from build123d import *

# Parameters (mm, degrees)
SKETCH1_R           = 12.5
SKETCH1_R_2         = 7.5
BOSS_EXTRUDE1_DEPTH = 15
SKETCH1_3_W         = 30
SKETCH1_3_H         = 15
BOSS_EXTRUDE2_DEPTH = 45
BOSS_EXTRUDE3_START = 15
SKETCH1_4_W         = 30
SKETCH1_4_H         = 15
BOSS_EXTRUDE3_DEPTH = 45
CUT_EXTRUDE1_START  = 10
SKETCH3_R           = 6
CUT_EXTRUDE1_DEPTH  = 30


with BuildPart() as part:
    # Sketch1 → Boss-Extrude1 (new body)
    with BuildSketch(Plane(origin=(0, 0, 0), x_dir=(1, 0, 0), z_dir=(0, 1, 0))):
        with BuildLine():
            Line((150, 25), (0, 25))
            ThreePointArc((0, 25), (-25, 0), (0, -25))
            Line((0, -25), (20, -25))
            Line((20, -25), (20, -10))
            Line((20, -10), (50, -10))
            Line((50, -10), (50, -25))
            Line((50, -25), (120, -25))
            Line((120, -25), (150, -25))
            Line((150, -25), (150, 25))
        make_face()
        with Locations(Location((0, 0, 0), (0, 0, 270))):
            Circle(SKETCH1_R, mode=Mode.SUBTRACT)
        with Locations(Location((135, 0, 0), (0, 0, 270))):
            Circle(SKETCH1_R_2, mode=Mode.SUBTRACT)
    extrude(amount=BOSS_EXTRUDE1_DEPTH)

    # Sketch1<3> → Boss-Extrude2 (add)
    with BuildSketch(Plane(origin=(0, 0, 0), x_dir=(1, 0, 0), z_dir=(0, 1, 0))):
        with Locations((35, -17.5)):
            Rectangle(SKETCH1_3_W, SKETCH1_3_H)
    extrude(amount=BOSS_EXTRUDE2_DEPTH)

    # Sketch1<4> → Boss-Extrude3 (add)
    with BuildSketch(Plane(origin=(0, 0, 0), x_dir=(1, 0, 0), z_dir=(0, 1, 0)).offset(BOSS_EXTRUDE3_START)):
        with Locations((135, -32.5)):
            Rectangle(SKETCH1_4_W, SKETCH1_4_H)
    extrude(amount=-BOSS_EXTRUDE3_DEPTH)

    # Sketch3 → Cut-Extrude1 (cut)
    with BuildSketch(Plane.XY.offset(CUT_EXTRUDE1_START)):
        with BuildLine():
            ThreePointArc((35, 45), (45.606601718, 40.606601718), (50, 30))
            Line((50, 30), (50, 45))
            Line((50, 45), (35, 45))
        make_face()
        with BuildLine():
            Line((20, 45), (20, 30))
            ThreePointArc((20, 30), (24.393398282, 40.606601718), (35, 45))
            Line((35, 45), (20, 45))
        make_face()
        with Locations(Location((35, 30, 0), (0, 0, 180))):
            Circle(SKETCH3_R)
        with BuildLine():
            ThreePointArc((150, -15), (135, -30), (120, -15))
            Line((120, -15), (120, -39.427079815))
            Line((120, -39.427079815), (150, -39.427079815))
            Line((150, -39.427079815), (150, -15))
        make_face()
        with Locations(Location((135, -15, 0), (0, 0, 180))):
            Circle(SKETCH3_R)
    extrude(amount=CUT_EXTRUDE1_DEPTH, mode=Mode.SUBTRACT)


solid = part.part
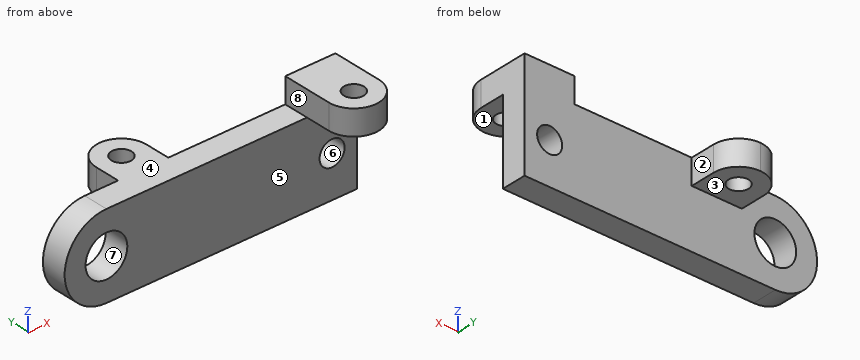
Build history of the part. All positions in model axes, mm. Face numbers are marked on the shaded views. A direction names the side the tool comes from. Round coordinates to 2 decimals unless told otherwise and drop trailing zeros. Write each loop counter-clockwise with the first axis right and the second up, starting at its lowest first coordinate (ties: lowest second). Pieces come first, ordered by that corner, then holes. Notation, with made-up numbers: M -14.75,-6.5 L 44.25,-6.5 A14 cw 44.25,4.5 Z; hole C 68,87.25 d4. An arc over 180 degrees is marked long. Answer as a JSON object with one key per item and string values. Group by question number.
(1) Cut at D-D (z = 19). Give the cut face in (x, y).
(2) Drill centre lines: L1, parallel to X at y = 8, z = 0; L2, parallel to Y at x = 135, z = 36; L3, parallel to X at y = -15, z = 34. Where is each one in solid material? Low to high.
(3) Cut at C-C (y = 8). Give the cut face in (x, z).
(4) Cut at B-B (x = 135). Give the cut face in (y, z), and give its area (3 significant figures).
(5) Which spindle directions (+Z, -Z, +X, -X, +Y, -Y) get a long thin tool onto all of the face, cutting with end or side? Do the marked faces 1, 2, 3 and 4. Say none if no direction does.
(6) Cut at A-A (z = 0). Give the cut face in (x, y).
(7) Mould opens along X. For the marked faces 5, 6, 7 and 8 say: pulls with the +X half, pulls with the -X half, needs draft (parallel to the pull), parting line crosses it, or undercut.
(8) Flat gauge pins, fed straight in: pin 1 (11 mm diameter, centred on x = 35, y = 30, fed in from -Z); pin 2 (5 mm diameter, centred on x = 78, z = 11, fed in from +Y); pin 3 (14 mm diameter, centred on x = 135, y = -15, fed in from +Z); pin 4 (16.5 mm diameter, centred on y = 23.5, z = 14.5, fed in from -X). Where does each tip first touch, or does it go through?
Responses:
{
 "1": {"outline": "M -16.25,0 L 150,0 L 150,15 L 50,15 L 50,30 A15 ccw 20,30 L 20,15 L -16.25,15 Z; hole C 35,30 d12"},
 "2": {"L1": "x = -25 to -12.5, 12.5 to 127.5, 142.5 to 150", "L2": "y = -30 to -21, -9 to 15", "L3": "x = 120 to 129, 141 to 150"},
 "3": {"outline": "M 0,-25 L 150,-25 L 150,40 L 120,40 L 120,25 L 0,25 A25 ccw Z; hole C 0,0 d25; hole C 135,0 d15"},
 "4": {"outline": "M -30,25 L -21,25 L -21,40 L -30,40 Z; M -9,25 L 0,25 L 0,7.5 L 15,7.5 L 15,40 L -9,40 Z; M 0,-25 L 15,-25 L 15,-7.5 L 0,-7.5 Z", "area": "1,020 mm2"},
 "5": {"face 1": "-Z, +X, -X, -Y", "face 2": "+Z, -Z, +X, +Y", "face 3": "-Z, +X, -X, +Y", "face 4": "+Z, -X, +Y, -Y"},
 "6": {"outline": "M -25,0 L -12.5,0 L -12.5,15 L -25,15 Z; M 12.5,0 L 127.5,0 L 127.5,15 L 12.5,15 Z; M 142.5,0 L 150,0 L 150,15 L 142.5,15 Z"},
 "7": {"face 5": "needs draft", "face 6": "undercut", "face 7": "undercut", "face 8": "pulls with the -X half"},
 "8": {"pin 1": "passes through", "pin 2": "stops at y = 15", "pin 3": "stops at z = 40", "pin 4": "stops at x = 20"}
}
